from build123d import *

# Parameters (mm, degrees)
F0_W      = 92
F0_H      = 18
F0_W_2    = 86.65
F0_H_2    = 14.25
F1_DEPTH  = 70
F2_DEPTH  = 35.8
F4_W      = 13.3
F4_H      = 8.6
F5_DEPTH  = 22
F3_R      = 2
F6_DEPTH  = 8
F8_DEPTH  = 4
F9_W      = 10.7813365757
F9_H      = 6.4464779571
F9_R      = 3.2
F10_DEPTH = 9.9
F11_W     = 4.2
F11_H     = 70
F12_DEPTH = 8.9
F13_R     = 4.9
F13_R_2   = 2.125
F14_DEPTH = 3.3
F15_DEPTH = 44.7


with BuildPart() as f1:
    # F0 (on Front) → F1 (new body)
    with BuildSketch(Plane.XZ):
        Rectangle(F0_W, F0_H)
        Rectangle(F0_W_2, F0_H_2, mode=Mode.SUBTRACT)
    extrude(amount=F1_DEPTH)

    # F0 (on Front) → F2 (join)
    with BuildSketch(Plane.XZ):
        Rectangle(F0_W_2, F0_H_2)
    extrude(amount=F2_DEPTH)

    # F4 (on face) → F5 (cut)
    with BuildSketch(Plane.XZ.offset(35.8)):
        Rectangle(F4_W, F4_H)
    extrude(amount=-F5_DEPTH, mode=Mode.SUBTRACT)

    # F3 (on Front) → F6 (cut)
    with BuildSketch(Plane.XZ):
        Circle(F3_R)
    extrude(amount=F6_DEPTH, mode=Mode.SUBTRACT)

    # F7 (on Front) → F8 (cut)
    with BuildSketch(Plane.XZ):
        with BuildLine():
            ThreePointArc((-16, -4.75), (-15.1945436483, -2.8054563517), (-13.25, -2))
            Line((-13.25, -2), (13.25, -2))
            ThreePointArc((13.25, -2), (15.1945436483, -2.8054563517), (16, -4.75))
            Line((16, -4.75), (16, -9.8020741716))
            Line((16, -9.8020741716), (20, -9.8020741716))
            Line((20, -9.8020741716), (20, -2))
            Line((20, -2), (20, -0.75))
            ThreePointArc((20, -0.75), (19.1945436483, 1.1945436483), (17.25, 2))
            Line((17.25, 2), (16, 2))
            Line((16, 2), (-16, 2))
            Line((-16, 2), (-17.25, 2))
            ThreePointArc((-17.25, 2), (-19.1945436483, 1.1945436483), (-20, -0.75))
            Line((-20, -0.75), (-20, -2))
            Line((-20, -2), (-20, -11.9064366445))
            Line((-20, -11.9064366445), (-16, -11.9064366445))
            Line((-16, -11.9064366445), (-16, -4.75))
        make_face()
    extrude(amount=F8_DEPTH, mode=Mode.SUBTRACT)

    # F9 (on face) → F10 (cut)
    with BuildSketch(Plane.XZ.offset(13.8)):
        with Locations((0, -0.695)):
            Rectangle(F9_W, F9_H)
        with Locations((0, -0.695)):
            Circle(F9_R, mode=Mode.SUBTRACT)
        with Locations((0, -0.695)):
            Circle(F9_R)
    extrude(amount=-F10_DEPTH, mode=Mode.SUBTRACT)

    # F11 (on face) → F12 (cut)
    with BuildSketch(Plane(origin=(0, 0, -9), x_dir=(1, 0, 0), z_dir=(0, 0, -1))):
        with Locations((0, 35)):
            Rectangle(F11_W, F11_H)
    extrude(amount=-F12_DEPTH, mode=Mode.SUBTRACT)

    # F13 (on face) → F14 (cut)
    with BuildSketch(Plane.XZ.offset(35.8)):
        with Locations((24.9875, 0)):
            Circle(F13_R)
        with Locations((24.9875, 0)):
            Circle(F13_R_2, mode=Mode.SUBTRACT)
        with Locations((-24.9875, 0)):
            Circle(F13_R)
        with Locations((-24.9875, 0)):
            Circle(F13_R_2, mode=Mode.SUBTRACT)
        with Locations((-24.9875, 0)):
            Circle(F13_R_2)
        with Locations((24.9875, 0)):
            Circle(F13_R_2)
    extrude(amount=-F14_DEPTH, mode=Mode.SUBTRACT)

    # F13 (on face) → F15 (cut)
    with BuildSketch(Plane.XZ.offset(35.8)):
        with Locations((-24.9875, 0)):
            Circle(F13_R_2)
        with Locations((24.9875, 0)):
            Circle(F13_R_2)
    extrude(amount=-F15_DEPTH, mode=Mode.SUBTRACT)


solid = f1.part
Geometry: final body of the model. Coordinates: model frame, mm. A direction names the side the tool comes from. Coordinates: 2 decimals unless noted, no trailing zeros. Loops run counter-clockwise (first coordinate to the right, second up) from the corner with the lowest first, then second, coordinate; pieces in that order, holes last. Notation, with made-up numbers: (26, -38.75) - (84, -38.75) arc R29 cw to (84, -14.75) - close; hole circle Ø4 at (54, -16). An arc over 180 degrees is marked (long way). One line per question, with ' | ' between items. Start each with the question number.
(1) Cut plane D-D on y = -62. Output: boundary loops of the cut face in (x, z) (3 decimals).
(2) Draft query along Z for faces 1 (the flat face through (20, -2, -5)), 2 (the flat face through (-4, -3.9, -3)), 3 (the flat face through (-24, -35, -9)). Return one class per face: +Z half, -Z half, draft (parallel to the pull), parting line (faces both ways), or undercut.
(3) Reachability of faces 4 (the flat face through (-4, -9, -3.918)), 5 (the flat face through (16, -2, -7)), 6 (the flat face through (-8, -2, -2)) from +Z, -Z, +X, -X, +Y, -Y: full face, straight path, thin tool, end or side. Return the list, or none.
(4) Cut plane B-B on y = -23. Count the separate pieces of the cut face and the enclosed holes in it, and give its area (3 significant figures).
(5) Cut plane A-A on x = 4. Output: boundary loops of the cut face in (y, z) (3 decimals), and give its area (3 significant figures).
(6) Cut plane C-C on x = 31. Output: boundary loops of the cut face in (y, z) (3 decimals), and give its area (3 significant figures).
(7) First-contact query: pin 1 (5 mm diameter, centred on x = 24, z = 1, fed in from -Y); pin 2 (1 mm diameter, centred on x = 3.5, z = -3, fed in from -Y). Flat tips, straight axial feed; report the tip coordinate or a pass-through.
(8) Ray query, L1, parallel to X at y = -66.5, z = 2.5 (3 decimals); L2, parallel to Z at x = 29, y = -65.5 (3 decimals); L3, parallel to X at y = -15.5, z = -7. Return the intervals inside material, ascending. Write a range as from..to.
Here are the results:
1) outline: (-46, -9) - (-2.1, -9) - (-2.1, -7.125) - (-43.325, -7.125) - (-43.325, 7.125) - (43.325, 7.125) - (43.325, -7.125) - (2.1, -7.125) - (2.1, -9) - (46, -9) - (46, 9) - (-46, 9) - close
2) face 1: draft | face 2: undercut | face 3: -Z half
3) face 4: -Y | face 5: -Z, +Y | face 6: +Y
4) separate pieces: 1 | enclosed holes: 2 | area: 1,490 mm²
5) outline: (-70, -9) - (0, -9) - (0, -2) - (-3.9, -2) - (-3.9, -3.918) - (-13.8, -3.918) - (-13.8, -4.3) - (-35.8, -4.3) - (-35.8, -7.125) - (-70, -7.125) - close; (-70, 7.125) - (-35.8, 7.125) - (-35.8, 4.3) - (-13.8, 4.3) - (-13.8, 2.528) - (-3.9, 2.528) - (-3.9, 2) - (0, 2) - (0, 9) - (-70, 9) - close | area: 504 mm²
6) outline: (-70, -9) - (0, -9) - (0, 9) - (-70, 9) - (-70, 7.125) - (-35.8, 7.125) - (-35.8, -7.125) - (-70, -7.125) - close | area: 773 mm²
7) pin 1: y = -32.5 | pin 2: y = -3.9
8) L1: -46..-43.325, 43.325..46 | L2: -9..-7.125, 7.125..9 | L3: -46..-2.1, 2.1..46
